CAD build for the part. Positions are in the model's coordinates, mm. Face numbers are marked on the shaded views. A direction names the side the tool comes from. Round coordinates to 2 decimals unless told otherwise and drop trailing zeros. Order: outer loops, then holes, each group sorted by start corner. A loop starts at its lowest first (then second) coordinate and runs counter-clockwise, first axis right, second up.
```python
from build123d import *

# Parameters (mm, degrees)
BOSS_EXTRU_1_DEPTH      = 70
ESQUISSE3_W             = 40
ESQUISSE3_H             = 16
ENL_V_MAT_EXTRU_1_DEPTH = 15
CONG_2_R                = 6
ESQUISSE4_W             = 58
ESQUISSE4_H             = 6
BOSS_EXTRU_2_DEPTH      = 30
ENL_V_MAT_EXTRU_2_REACH = 80.655
ESQUISSE5_R             = 2.1
ESQUISSE6_R             = 3.55
ENL_V_MAT_EXTRU_3_DEPTH = 4.2
ESQUISSE8_W             = 15.2
ESQUISSE8_H             = 4
ENL_V_MAT_EXTRU_5_DEPTH = 35
ENL_V_MAT_EXTRU_6_REACH = 80.119
ESQUISSE9_R             = 2.1
ESQUISSE10_W            = 3
ESQUISSE10_H            = 15
BOSS_EXTRU_3_DEPTH      = 22
CONG_3_R                = 3
CONG_4_R                = 4


with BuildPart() as part:
    # Esquisse1 → Boss.-Extru.1 (new body)
    with BuildSketch(Plane.XY):
        with BuildLine():
            Line((-16.668973791, 33.181519274), (-16.668973791, 15.181519274))
            Line((-16.668973791, 15.181519274), (-1.668973791, 15.181519274))
            Line((-1.668973791, 15.181519274), (-1.668973791, 21.181519274))
            Line((-1.668973791, 21.181519274), (-9.668973791, 21.181519274))
            ThreePointArc((-9.668973791, 21.181519274), (-12.497400916, 22.35309215), (-13.668973791, 25.181519274))
            Line((-13.668973791, 25.181519274), (-13.668973791, 31.181519274))
            Line((-13.668973791, 31.181519274), (-8.668973791, 35.681519274))
            ThreePointArc((-8.668973791, 35.681519274), (-9.108313619, 36.742179446), (-10.168973791, 37.181519274))
            Line((-10.168973791, 37.181519274), (-13.668973791, 37.181519274))
            Line((-13.668973791, 37.181519274), (-14.668973791, 37.181519274))
            Line((-14.668973791, 37.181519274), (-16.668973791, 37.181519274))
            Line((-16.668973791, 37.181519274), (-16.668973791, 34.181519274))
            Line((-16.668973791, 34.181519274), (-16.668973791, 33.181519274))
        make_face()
    extrude(amount=BOSS_EXTRU_1_DEPTH)

    # Esquisse3 → Enlèv. mat.-Extru.1 (cut)
    with BuildSketch(Plane.ZY.offset(16.668973791)):
        with Locations((35, 29.181519274)):
            Rectangle(ESQUISSE3_W, ESQUISSE3_H)
    extrude(amount=-ENL_V_MAT_EXTRU_1_DEPTH, mode=Mode.SUBTRACT)

    # Congé2
    cong_2_edges = [part.edges().sort_by_distance(p)[0] for p in [
        (-1.668973791, 18.181519274, 0),
        (-1.668973791, 18.181519274, 70),
    ]]
    fillet(cong_2_edges, radius=CONG_2_R)

    # Esquisse4 → Boss.-Extru.2 (add)
    with BuildSketch(Plane(origin=(-1.668973791, 0, 0), x_dir=(0, 0, -1), z_dir=(1, 0, 0))):
        with Locations((-35, 18.181519274)):
            Rectangle(ESQUISSE4_W, ESQUISSE4_H)
    extrude(amount=BOSS_EXTRU_2_DEPTH)

    # Esquisse5 → Enlèv. mat.-Extru.2 (cut, up to next)
    with BuildSketch(Plane.XZ.offset(-15.181519274), mode=Mode.PRIVATE) as enl_v_mat_extru_2_sk1:
        with Locations(Location((5.831026209, 39.5, 0), (0, 0, 270))):
            Circle(ESQUISSE5_R)
    enl_v_mat_extru_2_tool1 = extrude(enl_v_mat_extru_2_sk1.sketch, amount=-ENL_V_MAT_EXTRU_2_REACH, mode=Mode.PRIVATE) & part.part
    # Esquisse5 → Enlèv. mat.-Extru.2 (cut, up to next)
    with BuildSketch(Plane.XZ.offset(-15.181519274), mode=Mode.PRIVATE) as enl_v_mat_extru_2_sk2:
        with Locations(Location((5.831026209, 30.5, 0), (0, 0, 270))):
            Circle(ESQUISSE5_R)
    enl_v_mat_extru_2_tool2 = extrude(enl_v_mat_extru_2_sk2.sketch, amount=-ENL_V_MAT_EXTRU_2_REACH, mode=Mode.PRIVATE) & part.part
    add(enl_v_mat_extru_2_tool1.solids().sort_by_distance((5.831026, 15.181519, 39.5))[0], mode=Mode.SUBTRACT)
    add(enl_v_mat_extru_2_tool2.solids().sort_by_distance((5.831026, 15.181519, 30.5))[0], mode=Mode.SUBTRACT)

    # Esquisse6 → Enlèv. mat.-Extru.3 (cut)
    with BuildSketch(Plane(origin=(0, 21.181519274, 0), x_dir=(1, 0, 0), z_dir=(0, 1, 0))):
        with Locations(Location((5.831026209, -30.5, 0), (0, 0, 270))):
            Circle(ESQUISSE6_R)
        with Locations(Location((5.831026209, -39.5, 0), (0, 0, 270))):
            Circle(ESQUISSE6_R)
    extrude(amount=-ENL_V_MAT_EXTRU_3_DEPTH, mode=Mode.SUBTRACT)

    # Esquisse8 → Enlèv. mat.-Extru.5 (cut)
    with BuildSketch(Plane(origin=(28.331026209, 0, 0), x_dir=(0, 0, -1), z_dir=(1, 0, 0))):
        with Locations((-54.4, 19.181519274)):
            Rectangle(ESQUISSE8_W, ESQUISSE8_H)
        with Locations((-15.6, 19.181519274)):
            Rectangle(ESQUISSE8_W, ESQUISSE8_H)
    extrude(amount=-ENL_V_MAT_EXTRU_5_DEPTH, mode=Mode.SUBTRACT)

    # Esquisse9 → Enlèv. mat.-Extru.6 (cut, up to next)
    with BuildSketch(Plane(origin=(0, 17.181519274, 0), x_dir=(1, 0, 0), z_dir=(0, 1, 0)), mode=Mode.PRIVATE) as enl_v_mat_extru_6_sk1:
        with Locations(Location((23.331026209, -15.604527367, 0), (0, 0, 180))):
            Circle(ESQUISSE9_R)
    enl_v_mat_extru_6_tool1 = extrude(enl_v_mat_extru_6_sk1.sketch, amount=-ENL_V_MAT_EXTRU_6_REACH, mode=Mode.PRIVATE) & part.part
    add(enl_v_mat_extru_6_tool1.solids().sort_by_distance((23.331026, 17.181519, 15.604527))[0], mode=Mode.SUBTRACT)

    # Esquisse10 → Boss.-Extru.3 (add)
    with BuildSketch(Plane.XZ.offset(-15.181519274)):
        with Locations((-18.168973791, 62.5)):
            Rectangle(ESQUISSE10_W, ESQUISSE10_H)
        with Locations((-18.168973791, 7.5)):
            Rectangle(ESQUISSE10_W, ESQUISSE10_H)
    extrude(amount=-BOSS_EXTRU_3_DEPTH)

    # Congé3
    cong_3_edges = [part.edges().sort_by_distance(p)[0] for p in [
        (-19.668973791, 26.181519274, 55),
        (-19.668973791, 26.181519274, 15),
    ]]
    fillet(cong_3_edges, radius=CONG_3_R - 0.0001)  # a hair under: the kernel refuses the full size

    # Congé4
    cong_4_edges = [part.edges().sort_by_distance(p)[0] for p in [
        (-19.668973791, 26.181519274, 70),
        (-19.668973791, 26.181519274, 0),
    ]]
    fillet(cong_4_edges, radius=CONG_4_R)


solid = part.part
```
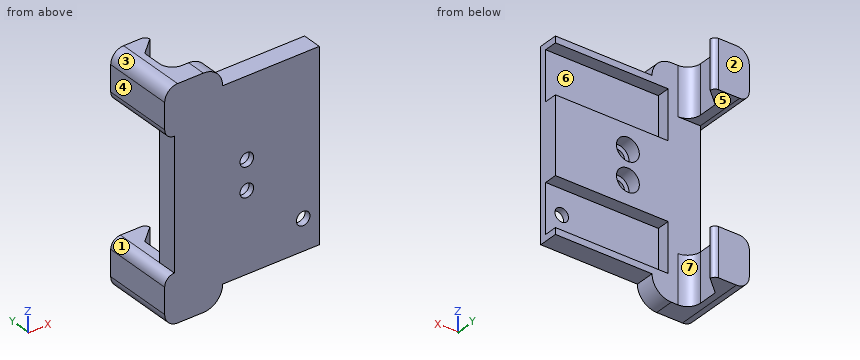
1. Tool access for the marked faces 4, 5, 6 and 7: list every direction of +Z, -Z, +X, -X, +Y, -Y with a clear straight run to the whole face (end or side of a thin tool).
2. Cut at D-D, the plane x = 15. Write the cut outline in (y, z).
3. Drill centre lines: line 1 (Z direction, x = -15.5, y = 31.75); line 2 (X direction, y = 16.5, z = 39.5); line 3 (Z direction, x = -3, y = 18.25). Where is each one in solid material? Low to high.
4. Cut at A-A, the plane y = 29.25. Write the cut outline in (x, z), and give its area (3 significant figures).
5. Pin check, flat tips, straight feed: P1, Ø6, axis at x = 6.5, z = 15, coming from the +Y side; P2, Ø10, axis at x = -6, y = 21, coming from the -Z side; P3, Ø2, axis at y = 19, z = 56, coming from the +X side; P4, Ø3, axis at y = 29.5, z = 11, coming from the +X side. Stop position of each tip, or through.
6. Cut at B-B, the plane z = 30.5. Write the cut outline in (x, y), and give its area (3 significant figures).
7. Cut at C-C, the plane x = -14.5. Write the cut outline in (y, z), and give its area (3 significant figures).
8. Mould opens along Z. For the marked faces 1, 2 and 3 say: released by +Z, released by -Z, zero draft, split by the parting line, or undercut.
Outcome:
1. face 4: +Z, -Z, -X, +Y, -Y
1. face 5: +X, -X, +Y
1. face 6: +X, +Y
1. face 7: +Z, -Z, +X
2. outline: (15.18, 6) - (21.18, 6) - (21.18, 8) - (17.18, 8) - (17.18, 23.2) - (21.18, 23.2) - (21.18, 46.8) - (17.18, 46.8) - (17.18, 62) - (21.18, 62) - (21.18, 64) - (15.18, 64) - close
3. line 1: z = 0 to 15, 55 to 70
3. line 2: x = -16.67 to 3.73, 7.93 to 28.33
3. line 3: z = 2.23 to 8, 23.2 to 46.8, 62 to 67.77
4. outline: (-19.67, 4) arc R4 ccw to (-15.67, 0) - (-13.67, 0) - (-13.67, 15) - (-16.67, 15) arc R3 ccw to (-19.67, 12) - close; (-19.67, 58) arc R3 ccw to (-16.67, 55) - (-13.67, 55) - (-13.67, 70) - (-15.67, 70) arc R4 ccw to (-19.67, 66) - close
4. area: 169 mm2
5. P1: stops at y = 17.18
5. P2: stops at z = 0
5. P3: stops at x = -6.67
5. P4: stops at x = -13.67
6. outline: (-16.67, 15.18) - (3.73, 15.18) - (3.73, 16.98) - (2.28, 16.98) - (2.28, 21.18) - (-16.67, 21.18) - close; (7.93, 15.18) - (28.33, 15.18) - (28.33, 21.18) - (9.38, 21.18) - (9.38, 16.98) - (7.93, 16.98) - close
6. area: 233 mm2
7. outline: (15.18, 0) - (37.18, 0) - (37.18, 15) - (21.18, 15) - (21.18, 55) - (37.18, 55) - (37.18, 70) - (15.18, 70) - close
7. area: 900 mm2
8. face 1: undercut
8. face 2: zero draft
8. face 3: released by +Z
